Job drawing, mm, ordinate dimensions from the low corner. One solid piece. A direction names the side the tool comes from. Round coordinates to 2 decimals unless told otherwise and drop trailing zeros. Loops run counter-clockwise (first coordinate to the right, second up) from the corner with the lowest first, then second, coordinate; pieces in that order, holes last. Notation, with made-up numbers: M -8.75,60.5 L 32.25,60.5 A27 ccw 32.25,99.5 Z; hole C 0,32.5 d11. An arc over 180 degrees is marked long. Put each result on its own line as item: value. Start each with the question number.
1) Drop flat-ended pins along their axis: pin 1 Ø2 at (x, z) = (4.5, 16.5) entering from -Y; pin 2 Ø8 at (x, z) = (7, 16) entering from -Y; pin 3 Ø12 at (y, z) = (4, 4) entering from +X. Give the stop position or say it passes through.
2) Slice it at A-A on x = 13.5. Give the cut face in (y, z) (1 decimal).
3) Which spindle directions (+Z, -Z, +X, -X, +Y, -Y) get a long thin tool onto all of the face, cutting with end or side? Do the marked faces 1 and 2. Say none if no direction does.
4) Slice it at B-B on y = 5.25. Give the cut face in (x, z) (1 decimal), then the cut area to 3 significant figures.
5) Slice it at D-D on y = 2.25. Give the cut face in (x, z) (1 decimal).
6) Probe line 1 along Z through (x, y) = (6, 18) (1 decimal); line 2 along X through (y, z) = (9, 5.25) (1 decimal); line 3 along Y through (x, z) = (16, 17.5) (1 decimal). List the from-to ranges inside material, lowest first.
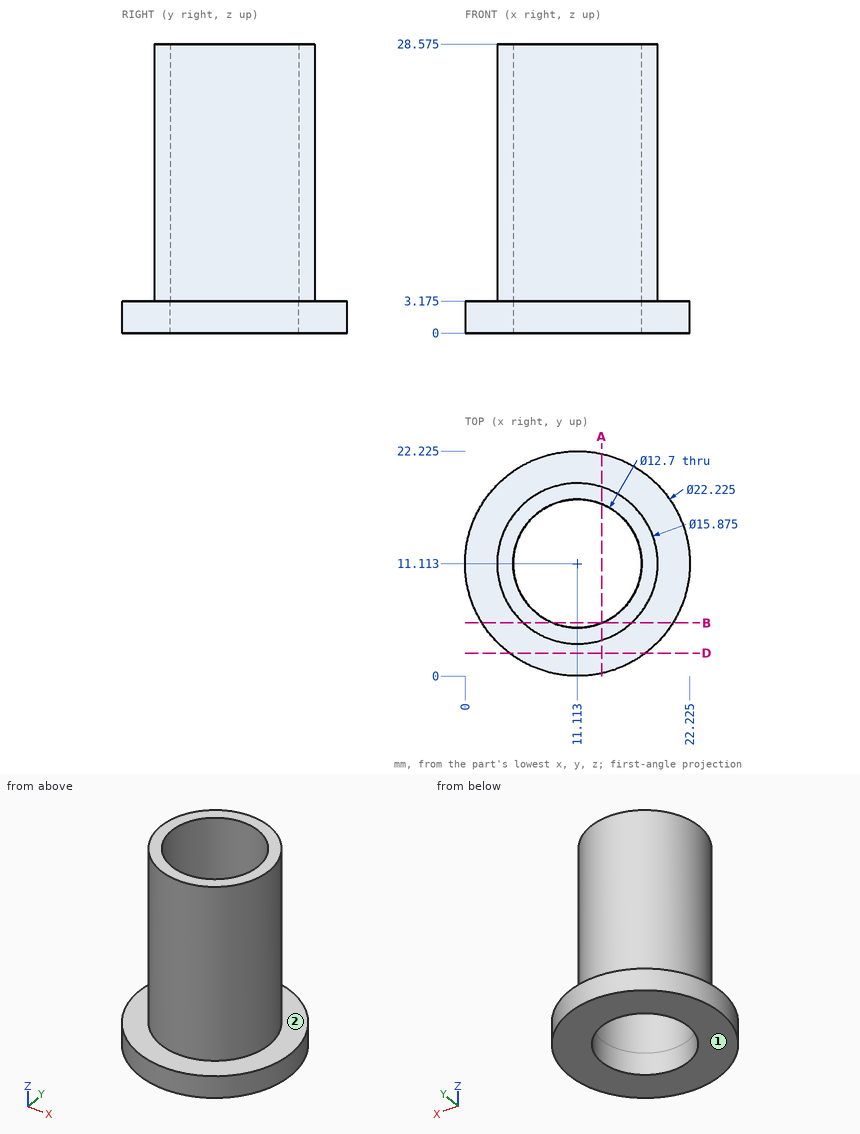
Recorded:
1. pin 1: stops at y = 5.5
1. pin 2: stops at y = 3.18
1. pin 3: stops at x = 22.16
2. outline: M 0.3,0 L 5.2,0 L 5.2,28.6 L 3.5,28.6 L 3.5,3.2 L 0.3,3.2 Z; M 17,0 L 22,0 L 22,3.2 L 18.7,3.2 L 18.7,28.6 L 17,28.6 Z
3. face 1: -Z, +X, -X, +Y, -Y
3. face 2: +Z
4. outline: M 1.7,0 L 8.7,0 L 8.7,28.6 L 5.8,28.6 L 5.8,3.2 L 1.7,3.2 Z; M 13.6,0 L 20.6,0 L 20.6,3.2 L 16.5,3.2 L 16.5,28.6 L 13.6,28.6 Z
4. area: 192 mm2
5. outline: M 4.4,0 L 17.8,0 L 17.8,3.2 L 4.4,3.2 Z
6. line 1: z = 0 to 3.2
6. line 2: x = 3.5 to 5.1, 17.1 to 18.8
6. line 3: y = 4.9 to 7.1, 15.2 to 17.4
